from build123d import *

# Parameters (mm, degrees)
F0_W      = 127
F0_H      = 25.4
F1_DEPTH  = 152.4
F2_W      = 106.8398617208
F2_H      = 12.6475254074
F3_DEPTH  = 152.401
F4_R      = 2.38125
F5_DEPTH  = 127.001
F6_R      = 2.38125
F7_DEPTH  = 127.001
F8_W      = 22.5498136133
F8_H      = 52.1139763296
F9_DEPTH  = 12.7534745926
F10_W     = 20.2880082652
F10_H     = 51.4018163085
F11_DEPTH = 12.7534745926
F12_W     = 65.1156418025
F12_H     = 21.9442248344
F13_DEPTH = 12.7534745926


with BuildPart() as f1:
    # F0 (on Front) → F1 (new body)
    with BuildSketch(Plane.XZ):
        with Locations((-5.044566528, 12.7)):
            Rectangle(F0_W, F0_H)
    extrude(amount=F1_DEPTH)

    # F2 (on face) → F3 (cut, through all)
    with BuildSketch(Plane.XZ.offset(152.4)):
        with Locations((-4.6506356448, 6.3237627037)):
            Rectangle(F2_W, F2_H)
    extrude(amount=-F3_DEPTH, mode=Mode.SUBTRACT)

    # F4 (on face) → F5 (cut, through all)
    with BuildSketch(Plane.YZ.offset(58.455433472)):
        with Locations((-16.5433734655, 8.7655037642)):
            Circle(F4_R)
    extrude(amount=-F5_DEPTH, mode=Mode.SUBTRACT)

    # F6 (on face) → F7 (cut, through all)
    with BuildSketch(Plane.YZ.offset(58.455433472)):
        with Locations((-144.9289917946, 5.8498084545)):
            Circle(F6_R)
    extrude(amount=-F7_DEPTH, mode=Mode.SUBTRACT)

    # F8 (on face) → F9 (cut, through all)
    with BuildSketch(Plane(origin=(0, 0, 12.6475254074), x_dir=(1, 0, 0), z_dir=(0, 0, -1))):
        with Locations((26.4765219763, 26.0569881648)):
            Rectangle(F8_W, F8_H)
    extrude(amount=-F9_DEPTH, mode=Mode.SUBTRACT)

    # F10 (on face) → F11 (cut, through all)
    with BuildSketch(Plane(origin=(0, 0, 12.6475254074), x_dir=(1, 0, 0), z_dir=(0, 0, -1))):
        with Locations((-31.5784798004, 25.7009081542)):
            Rectangle(F10_W, F10_H)
    extrude(amount=-F11_DEPTH, mode=Mode.SUBTRACT)

    # F12 (on face) → F13 (cut, through all)
    with BuildSketch(Plane(origin=(0, 0, 12.6475254074), x_dir=(1, 0, 0), z_dir=(0, 0, -1))):
        with Locations((-3.3583734185, 121.5704679489)):
            Rectangle(F12_W, F12_H)
    extrude(amount=-F13_DEPTH, mode=Mode.SUBTRACT)


solid = f1.part
Model file for the job. Use its own axes, mm. A direction names the side the tool comes from. Give positions to 0.01 mm unless a question says otherwise; leave off trailing zeros. Loops run counter-clockwise (first coordinate to the right, second up) from the corner with the lowest first, then second, coordinate; pieces in that order, holes last. Notation, with made-up numbers: (30, 53.25) -> (76, 53.25) arc R28 ccw to (76, 76.25) -> close; hole circle Ø10 at (-6, -14.5). An arc over 180 degrees is marked (long way). Use a Markdown table: item, result. Add a question column.
(1) Wall check: line 1 along X through (y, z) = (-23, 19.5); line 2 along X through (y, z) = (-43, 5); line 3 along Y through (x, z) = (22, 16.5). Give the ranges that are in metal, low to high.
(2) Slice it at D-D on y = -67. List the corners of the cut face in (x, z), and give its area (3 significant figures).
(3) Slice it at B-B on y = -44.5. List the corners of the cut face in (x, z).
(4) Tool access for faces 4 (the flat face through (-3, 0, 19)), 5 (the flat face through (-4, -132.543, 19)), 6 (the flat face through (-5, -77, 12.648)), 7 (the flat face through (-6, -152.4, 16)), 8 (the flat face through (37.751, -26, 19)): list every direction of +Z, -Z, +X, -X, +Y, -Y with a clear straight run to the whole face (end or side of a thin tool).
(5) Mould opens along Z. For faces 1 (the flat face through (29.199, -121, 19)), 2 (the cylindrical face through (-63.23, -14.27, 9.48)), 3 (the flat face through (-63, -75, 0)) say: +Z half, -Z half, draft (parallel to the pull), parting line (faces both ways), or undercut.
(6) Drop flat-ended pins along their axis: pin 1 Ø4 at (x, z) = (23, 11.5) entering from +Y; pin 2 Ø3 at (x, z) = (28, 10.5) entering from +Y; pin 3 Ø5.5 at (y, z) = (-16.54, 8.77) entering from -X; pin 4 Ø6 at (x, y) = (-44, -129) entering from -Z. Give the stop position or say it passes through.
(7) Slice it at A-A on x = 1.5. List the corners of the cut face in (y, z), and give its area (3 significant figures).
(8) Slice it at C-C on z = 17.25. List the corners of the cut face in (x, y).
Filled sheet:
| question | item | result |
|---|---|---|
| 1 | line 1 | -68.54 to -41.72, -21.43 to 15.2, 37.75 to 58.46 |
| 1 | line 2 | -68.54 to -58.07, 48.77 to 58.46 |
| 1 | line 3 | -152.4 to -132.54, -110.6 to -52.11 |
| 2 | outline | (-68.54, 0) -> (-58.07, 0) -> (-58.07, 12.65) -> (48.77, 12.65) -> (48.77, 0) -> (58.46, 0) -> (58.46, 25.4) -> (-68.54, 25.4) -> close |
| 2 | area | 1,870 mm2 |
| 3 | outline | (-68.54, 0) -> (-58.07, 0) -> (-58.07, 12.65) -> (-41.72, 12.65) -> (-41.72, 25.4) -> (-68.54, 25.4) -> close; (-21.43, 12.65) -> (15.2, 12.65) -> (15.2, 25.4) -> (-21.43, 25.4) -> close; (37.75, 12.65) -> (48.77, 12.65) -> (48.77, 0) -> (58.46, 0) -> (58.46, 25.4) -> (37.75, 25.4) -> close |
| 4 | face 4 | +Z, -Z, +X, -X, +Y |
| 4 | face 5 | +Z, -Z |
| 4 | face 6 | -Z, +Y, -Y |
| 4 | face 7 | +Z, -Z, +X, -X, -Y |
| 4 | face 8 | +Z, -Z, +Y |
| 5 | face 1 | draft |
| 5 | face 2 | undercut |
| 5 | face 3 | -Z half |
| 6 | pin 1 | y = -52.11 |
| 6 | pin 2 | through |
| 6 | pin 3 | x = -68.54 |
| 6 | pin 4 | z = 12.65 |
| 7 | outline | (-152.4, 12.65) -> (-132.54, 12.65) -> (-132.54, 25.4) -> (-152.4, 25.4) -> close; (-110.6, 12.65) -> (0, 12.65) -> (0, 25.4) -> (-110.6, 25.4) -> close |
| 7 | area | 1,660 mm2 |
| 8 | outline | (-68.54, -152.4) -> (58.46, -152.4) -> (58.46, 0) -> (37.75, 0) -> (37.75, -52.11) -> (15.2, -52.11) -> (15.2, 0) -> (-21.43, 0) -> (-21.43, -51.4) -> (-41.72, -51.4) -> (-41.72, 0) -> (-68.54, 0) -> close; hole (-35.92, -132.54) -> (29.2, -132.54) -> (29.2, -110.6) -> (-35.92, -110.6) -> close |
